Answer from the drawing. Dimensions are ordinates in mm from the lowest x, y and z of the part. Coordinates: 2 decimals unless noted, no trailing zeros. Write each loop counter-clockwise with the first axis right and the second up, starting at its lowest first coordinate (ties: lowest second). Pieces come first, ordered by that corner, then holes.
(1) The part is cut by section A-A on x = 93. Determine the outline of the cut face in (y, z) (1 decimal).
(2) The part is cut by section B-B on y = 22.5. Determine the outline of the cut face in (x, z).
(3) The part is cut by section C-C on z = 39. Determine the outline of the cut face in (x, y) (1 decimal), plus the area to 3 significant figures.
(4) Straight lines are drawn through the part: line 1 (Y direction, x = 102, z = 130) (1 decimal); line 2 (Z direction, x = 131.5, y = 38). For each, find the intervals that lie inside material, in ascending order.
(5) For a pull along Y with two mould halves and no side action, classify the marked faces 1, 2 and 3 as +Y half, -Y half, draft (parallel to the pull), parting line (faces both ways), or undercut.
(6) Given P1, Ø2, axis at x = 69.5, y = 21, coming from the -Z side; P2, Ø4.5, axis at x = 7.86, z = 12.52, coming from the -Y side; P3, Ø3.5, axis at x = 80, y = 74.5, coming from the +Z side; P4, Ø10, axis at x = 7.86, z = 168.1, coming from the -Y side (3 decimals), each flat-ended and moving along its own axis, determine where each tip first touches the part or whether it passes through.
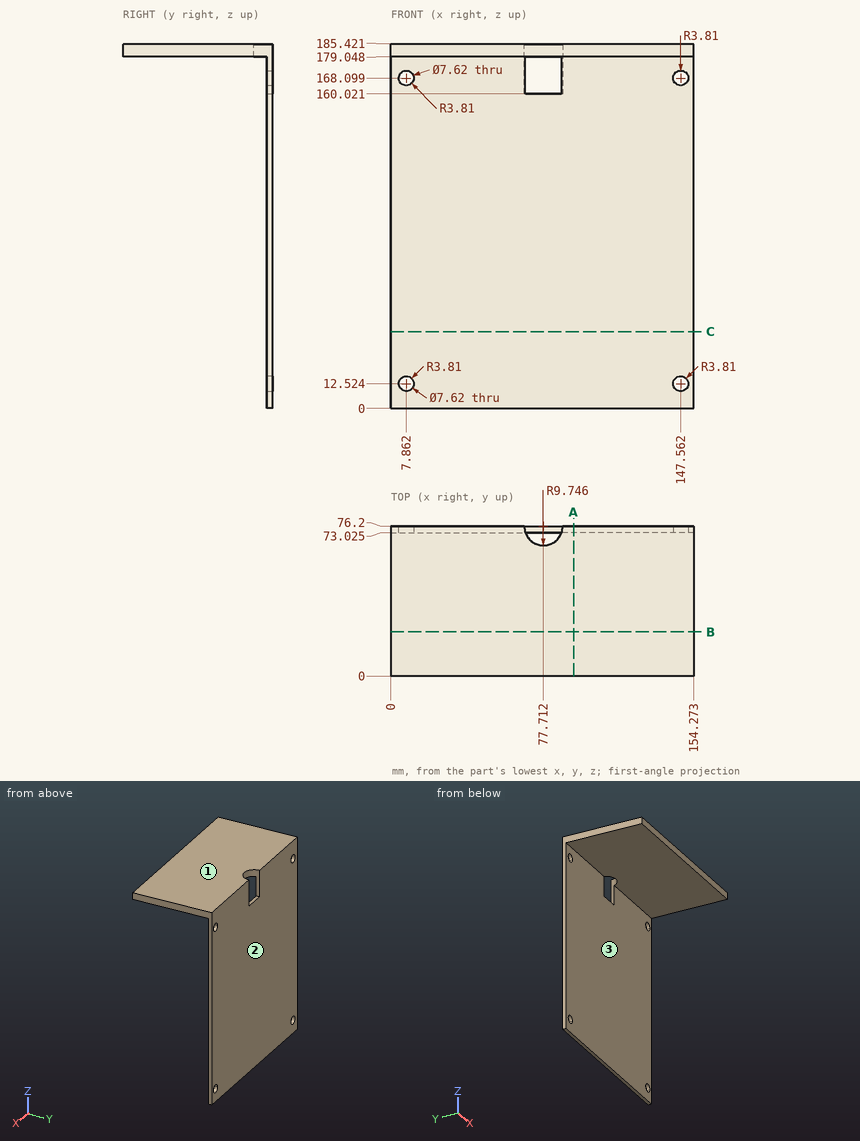
Model answer:
1. outline: (0, 179) - (73, 179) - (73, 0) - (76.2, 0) - (76.2, 185.4) - (0, 185.4) - close
2. outline: (0, 179.05) - (154.27, 179.05) - (154.27, 185.42) - (0, 185.42) - close
3. outline: (0, 73) - (154.3, 73) - (154.3, 76.2) - (0, 76.2) - close
3. area: 490 mm2
4. line 1: y = 73 to 76.2
4. line 2: z = 179.05 to 185.42
5. face 1: draft
5. face 2: +Y half
5. face 3: -Y half
6. P1: stops at z = 179.05
6. P2: passes through
6. P3: stops at z = 160.02
6. P4: stops at y = 73.025
